```python
from build123d import *

# Parameters (mm, degrees)
SKETCH1_R           = 1.5
SKETCH1_R_2         = 4.5
SKETCH1_W           = 99
SKETCH1_H           = 41
BOSS_EXTRUDE1_DEPTH = 3


with BuildPart() as part:
    # Sketch1 → Boss-Extrude1 (new body)
    with BuildSketch(Plane(origin=(0, 0, 0), x_dir=(1, 0, 0), z_dir=(0, 1, 0))):
        with BuildLine():
            Line((69.094938721, -38.021047238), (69.094938721, 11.978952762))
            ThreePointArc((69.094938721, 11.978952762), (66.166006532, 19.050020574), (59.094938721, 21.978952762))
            Line((59.094938721, 21.978952762), (-56.968320128, 21.978952762))
            ThreePointArc((-56.968320128, 21.978952762), (-64.039387939, 19.050020574), (-66.968320128, 11.978952762))
            Line((-66.968320128, 11.978952762), (-66.968320128, -38.021047238))
            ThreePointArc((-66.968320128, -38.021047238), (-64.039387939, -45.09211505), (-56.968320128, -48.021047238))
            Line((-56.968320128, -48.021047238), (59.094938721, -48.021047238))
            ThreePointArc((59.094938721, -48.021047238), (66.166006532, -45.09211505), (69.094938721, -38.021047238))
        make_face()
        with Locations((-58.93171984, 14.978952762)):
            Circle(SKETCH1_R, mode=Mode.SUBTRACT)
        with Locations((34.06828016, 14.978952762)):
            Circle(SKETCH1_R, mode=Mode.SUBTRACT)
        with Locations((-58.93171984, -40.021047238)):
            Circle(SKETCH1_R, mode=Mode.SUBTRACT)
        with Locations((34.06828016, -40.021047238)):
            Circle(SKETCH1_R, mode=Mode.SUBTRACT)
        with Locations((43.96828016, 5.978952762)):
            Circle(SKETCH1_R_2, mode=Mode.SUBTRACT)
        with Locations((-12.43171984, -12.521047238)):
            Rectangle(SKETCH1_W, SKETCH1_H, mode=Mode.SUBTRACT)
    extrude(amount=BOSS_EXTRUDE1_DEPTH)


solid = part.part
```
Design review of the part built by this model. Coordinates are the model's own, in mm. A direction names the side the tool comes from. Coordinates: 2 decimals unless noted, no trailing zeros. Order: outer loops, then holes, each group sorted by start corner. A loop starts at its lowest first (then second) coordinate and runs counter-clockwise, first axis right, second up. Notation, with made-up numbers: (15, -13) - (50, -13) arc R4 ccw to (50, -7) - close; hole circle Ø1 at (87, 6). An arc over 180 degrees is marked (long way). Answer in a Markdown table with one row per item.
(1) For faces 5 (the flat face through (15, 0, 36)), 6 (the flat face through (-13, 1, 33.021)), list the 3-axis set-ups (+Z, -Z, +X, -X, +Y, -Y) from which the entire face can be reached by the end or side of a thin tool; tool diameter is ignored.
Checked values:
| item | result |
|---|---|
| face 5 | +Z, -Z, +X, -X, -Y |
| face 6 | +Y, -Y |
(2) The part is to be moulded in two halves that separate along X. For faces 1 (the flat face through (-13, 1, -7.979)), 2 (the flat face through (15, 3, 36)), 3 (the flat face through (69.095, 1, 13)), 4 (the cylindrical face through (34.875, 1.479, -16.244)), say which applies: released by +X, released by -X, zero draft, split by the parting line, or undercut.
Checked values:
| item | result |
|---|---|
| face 1 | undercut |
| face 2 | zero draft |
| face 3 | released by +X |
| face 4 | undercut |
(3) Consider section B-B on x = -40. State the section outline as (y, z) points, plus the area to 3 significant figures.
Checked values:
| item | result |
|---|---|
| outline | (0, -21.98) - (3, -21.98) - (3, -7.98) - (0, -7.98) - close; (0, 33.02) - (3, 33.02) - (3, 48.02) - (0, 48.02) - close |
| area | 87.0 mm^2 |
(4) Consider section A-A on z = 24. State the section outline as (x, y) points.
Checked values:
| item | result |
|---|---|
| outline | (-66.97, 0) - (-61.93, 0) - (-61.93, 3) - (-66.97, 3) - close; (37.07, 0) - (69.09, 0) - (69.09, 3) - (37.07, 3) - close |
(5) Wall thickness on line 1 along Z through (x, y) = (29, 2.6); line 2 along X through (y, z) = (1.5, 19); line 3 along X through (y, z) = (2.25, -7): over which ranges is each line inside the solid? List them lowest first. Write a range as from..to.
Checked values:
| item | result |
|---|---|
| line 1 | -21.98..-7.98, 33.02..48.02 |
| line 2 | -66.97..-61.93, 37.07..69.09 |
| line 3 | -66.97..-61.93, 37.07..39.59, 48.35..69.09 |
(6) Consider section C-C on y = 2.55. State the section outline as (x, z) points.
Checked values:
| item | result |
|---|---|
| outline | (-66.97, -11.98) arc R10 ccw to (-56.97, -21.98) - (59.09, -21.98) arc R10 ccw to (69.09, -11.98) - (69.09, 38.02) arc R10 ccw to (59.09, 48.02) - (-56.97, 48.02) arc R10 ccw to (-66.97, 38.02) - close; hole (-61.93, -7.98) - (37.07, -7.98) - (37.07, 33.02) - (-61.93, 33.02) - close; hole circle Ø3 at (-58.93, -14.98); hole circle Ø3 at (-58.93, 40.02); hole circle Ø3 at (34.07, -14.98); hole circle Ø3 at (34.07, 40.02); hole circle Ø9 at (43.97, -5.98) |
